Here's how the part is built. I have some questions about the finished solid (model axes, mm). A direction names the side the tool comes from. Give positions to 0.01 mm unless a question says otherwise; leave off trailing zeros. Order: outer loops, then holes, each group sorted by start corner. A loop starts at its lowest first (then second) coordinate and runs counter-clockwise, first axis right, second up. Notation, with made-up numbers: (89, 55.5) - (105, 55.5) arc R10 ccw to (105, 73.5) - close; hole circle Ø9 at (-22, 45). An arc over 180 degrees is marked (long way). One line per question, with ' | ' between items.
from build123d import *

# Parameters (mm, degrees)
BOSS_EXTRUDE1_DEPTH = 4
BOSS_EXTRUDE2_DEPTH = 3
SKETCH4_R           = 4.5
CUT_EXTRUDE2_DEPTH  = 121.411793442


with BuildPart() as part:
    # Sketch1 → Boss-Extrude1 (new body)
    with BuildSketch(Plane(origin=(0, 0, 0), x_dir=(1, 0, 0), z_dir=(0, 1, 0))):
        with BuildLine():
            Line((-77, 85), (77, 85))
            ThreePointArc((77, 85), (82.656854249, 82.656854249), (85, 77))
            Line((85, 77), (85, -77))
            ThreePointArc((85, -77), (82.656854249, -82.656854249), (77, -85))
            Line((77, -85), (-77, -85))
            ThreePointArc((-77, -85), (-82.656854249, -82.656854249), (-85, -77))
            Line((-85, -77), (-85, 77))
            ThreePointArc((-85, 77), (-82.656854249, 82.656854249), (-77, 85))
        make_face()
    extrude(amount=BOSS_EXTRUDE1_DEPTH)

    # Sketch2 → Boss-Extrude2 (add)
    with BuildSketch(Plane.XZ):
        with BuildLine():
            Line((77, 82), (-77, 82))
            ThreePointArc((-77, 82), (-80.535533906, 80.535533906), (-82, 77))
            Line((-82, 77), (-82, -77))
            ThreePointArc((-82, -77), (-80.535533906, -80.535533906), (-77, -82))
            Line((-77, -82), (77, -82))
            ThreePointArc((77, -82), (80.535533906, -80.535533906), (82, -77))
            Line((82, -77), (82, 77))
            ThreePointArc((82, 77), (80.535533906, 80.535533906), (77, 82))
        make_face()
        with BuildLine():
            ThreePointArc((79, 77), (78.414213562, 78.414213562), (77, 79))
            Line((77, 79), (-77, 79))
            ThreePointArc((-77, 79), (-78.414213562, 78.414213562), (-79, 77))
            Line((-79, 77), (-79, -77))
            ThreePointArc((-79, -77), (-78.414213562, -78.414213562), (-77, -79))
            Line((-77, -79), (77, -79))
            ThreePointArc((77, -79), (78.414213562, -78.414213562), (79, -77))
            Line((79, -77), (79, 77))
        make_face(mode=Mode.SUBTRACT)
    extrude(amount=BOSS_EXTRUDE2_DEPTH)

    # Sketch4 → Cut-Extrude2 (cut, through all)
    with BuildSketch(Plane.XZ.offset(3)):
        with Locations(Location((77, 77, 0), (0, 0, 270))):
            Circle(SKETCH4_R)
        with Locations(Location((77, -77, 0), (0, 0, 270))):
            Circle(SKETCH4_R)
        with Locations(Location((-77, -77, 0), (0, 0, 270))):
            Circle(SKETCH4_R)
        with Locations(Location((-77, 77, 0), (0, 0, 270))):
            Circle(SKETCH4_R)
    extrude(amount=-CUT_EXTRUDE2_DEPTH, mode=Mode.SUBTRACT)


solid = part.part
1) I want a section at A-A (x = -65). List the corners of the cut face in (y, z) for me.
Model answer:
outline: (-3, -82) - (0, -82) - (0, -85) - (4, -85) - (4, 85) - (0, 85) - (0, 82) - (-3, 82) - (-3, 79) - (0, 79) - (0, -79) - (-3, -79) - close
2) I'm going to push flat-ended pins straight in: P1, Ø0.9, axis at y = -1, z = -17, coming from the -X side; P2, Ø1.5, axis at x = -2, y = -1.5, coming from the -Z side; P3, Ø14.5, axis at x = 77, z = 77, coming from the +Y side; P4, Ø0.9, axis at x = 25, y = -1.5, coming from the +Z side. Where does each tip first touch, or does it pass through?
Model answer:
P1: stops at x = -82 | P2: stops at z = -82 | P3: stops at y = 4 | P4: stops at z = 82
3) On a 3-axis mill with a long thin cutter (end or side, diameter ignored), from which of +Z, -Z, +X, -X, +Y, -Y can I reach the whole of each face in a straight line? I mean faces 5 (the face through (81, -1, 80)), 6 (the face through (-80, -1, 81)), 7 (the face through (1, 4, -1)), 8 (the face through (80, -1, -81)), 9 (the face through (1, 0, -1)). Say none if no direction works.
Model answer:
face 5: +Z, +X, -Y | face 6: +Z, -X, -Y | face 7: +Z, -Z, +X, -X, +Y | face 8: -Z, +X, -Y | face 9: -Y
4) I want a section at B-B (z = -58). List the corners of the cut face in (x, y) for me.
Model answer:
outline: (-85, 0) - (-82, 0) - (-82, -3) - (-79, -3) - (-79, 0) - (79, 0) - (79, -3) - (82, -3) - (82, 0) - (85, 0) - (85, 4) - (-85, 4) - close
5) Please list where these lines run through material, in increasing order: L1, parallel to Z at x = -77, y = 0.25; L2, parallel to X at y = -1.5, z = -77.
Model answer:
L1: z = -85 to -81.5, -72.5 to 72.5, 81.5 to 85 | L2: x = -82 to -81.5, 81.5 to 82
6) Thinking about a two-plate mould opening in X: for faces 1 (the face through (80.794, 0.451, -79.419)), 2 (the face through (85, 2, -1)), 3 (the face through (1, 2, 85)), 4 (the face through (-85, 2, 1)), which applies, +X half, -X half, draft (parallel to the pull), parting line (faces both ways), or undercut?
Model answer:
face 1: undercut | face 2: +X half | face 3: draft | face 4: -X half
